Geometry: final body of the model. Coordinates: model frame, mm. A direction names the side the tool comes from. Round coordinates to 2 decimals unless told otherwise and drop trailing zeros. Loops run counter-clockwise (first coordinate to the right, second up) from the corner with the lowest first, then second, coordinate; pieces in that order, holes last. Notation, with made-up numbers: (65, 9.5) -> (114, 9.5) arc R13 cw to (114, 25.5) -> close; hole circle Ø5 at (17.25, 11). An arc over 180 degrees is marked (long way). Answer in a Markdown table with one row per item.
Autodesk Inventor part; units mm, degrees
ref_plane "YZ Plane" through (0, 0, 0) normal (1, 0, 0) x (0, 1, 0)
ref_plane "XZ Plane" through (0, 0, 0) normal (0, 1, 0) x (-1, 0, 0)
ref_plane "XY Plane" through (0, 0, 0) normal (0, 0, 1) x (1, 0, 0)
sketch "Sketch1" plane through (0, 0, 0) normal (0, 1, 0) x (-1, 0, 0)
  line L0 (-42.5, 49) -> (42.5, 49)
  line L1 (42.5, 49) -> (42.5, -49)
  line L2 (42.5, -49) -> (-42.5, -49)
  line L3 (-42.5, -49) -> (-42.5, 49)
  line L4 (-42.5, 49) -> (42.5, -49) construction
  line L5 (42.5, 49) -> (-42.5, -49) construction
  line L6 (-39, 44) -> (39, 44) construction
  line L7 (39, 44) -> (39, -44) construction
  line L8 (39, -44) -> (-39, -44) construction
  line L9 (-39, -44) -> (-39, 44) construction
  line L10 (-39, 44) -> (39, -44) construction
  line L11 (39, 44) -> (-39, -44) construction
  point P0 (0, 0)
  dimension "d0" = 85
  dimension "d1" = 98
  dimension "d2" = 78
  dimension "d3" = 88
extrude "Extrusion1" add sketch "Sketch1" along normal blind 2
hole "Hole1" at (39, 0, 44) at (39, 0, -44) at (-39, 0, -44) at (-39, 0, 44) direction (0, 1, 0) diameter 3.6 end through all
sketch "Sketch2" plane through (0, 2, 0) normal (0, 1, 0) x (1, 0, 0)
  line L0 (40, -40) -> (-40, -40)
  line L1 (-40, -40) -> (-40, 40)
  line L2 (-40, 40) -> (40, 40)
  line L3 (40, 40) -> (40, -40)
  line L4 (40, -40) -> (-40, 40) construction
  line L5 (-40, -40) -> (40, 40) construction
  point P0 (0, 0)
  dimension "d13" = 80
  dimension "d14" = 80
extrude "Extrusion2" add sketch "Sketch2" along normal blind 10
properties part number "mainboard"
Item 1: Section query D-D, the plane z = 21. Output: boundary loops of the cut face in (x, y).
Ans:
| item | result |
|---|---|
| outline | (-42.5, 0) -> (42.5, 0) -> (42.5, 2) -> (40, 2) -> (40, 12) -> (-40, 12) -> (-40, 2) -> (-42.5, 2) -> close |
Item 2: Set-up query: faces 1 (the flat face through (-1, 7, -40)), 2 (the flat face through (40, 7, -1)), 3 (the flat face through (-40, 7, 1)), 4 (the flat face through (1, 7, 40)). Return all of +Z, -Z, +X, -X, +Y, -Y with unobstructed straight access to the full face (end or side cutting, diameter ignored); none if empty.
Ans:
| item | result |
|---|---|
| face 1 | -Z, +X, -X, +Y |
| face 2 | +Z, -Z, +X, +Y |
| face 3 | +Z, -Z, -X, +Y |
| face 4 | +Z, +X, -X, +Y |
Item 3: Section query A-A, the plane z = 44. Output: boundary loops of the cut face in (x, y).
Ans:
| item | result |
|---|---|
| outline | (-42.5, 0) -> (-40.8, 0) -> (-40.8, 2) -> (-42.5, 2) -> close; (-37.2, 0) -> (37.2, 0) -> (37.2, 2) -> (-37.2, 2) -> close; (40.8, 0) -> (42.5, 0) -> (42.5, 2) -> (40.8, 2) -> close |
Item 4: Section query C-C, the plane y = 5.5. Output: boundary loops of the cut face in (x, z).
Ans:
| item | result |
|---|---|
| outline | (-40, -40) -> (40, -40) -> (40, 40) -> (-40, 40) -> close |
Item 5: First-contact query: P1, Ø4, axis at x = 4.5, y = 5, coming from the -Z side; P2, Ø2, axis at x = 26.5, z = 32.5, coming from the -Y side; P3, Ø5, axis at x = 15, y = 5, coming from the +Z side; P4, Ø5, axis at y = 6, z = 2.5, coming from the +X side. Flat tips, straight axial feed; report the tip coordinate or a pass-through.
Ans:
| item | result |
|---|---|
| P1 | z = -40 |
| P2 | y = 0 |
| P3 | z = 40 |
| P4 | x = 40 |
Item 6: Mould query, pull axis X, two halves, no side actions, for faces 5 (the cylindrical face through (-40.785, 1.014, 44.234)), 6 (the flat face through (0.2, 2, 40.2)), 7 (the flat face through (42.5, 1, -1)). Classes: released by +X, released by -X, zero draft, split by the parting line, or undercut.
Ans:
| item | result |
|---|---|
| face 5 | undercut |
| face 6 | zero draft |
| face 7 | released by +X |
Item 7: Ray query, L1, parallel to Z at x = 39, y = 1.4; L2, parallel to X at y = 0.95, z = 44; L3, parallel to Z at x = -8, y = 11.25. Return the intervals inside material, ascending.
Ans:
| item | result |
|---|---|
| L1 | -49 to -45.8, -42.2 to 42.2, 45.8 to 49 |
| L2 | -42.5 to -40.8, -37.2 to 37.2, 40.8 to 42.5 |
| L3 | -40 to 40 |
Item 8: Section query B-B, the plane x = 4. Output: boundary loops of the cut face in (y, z).
Ans:
| item | result |
|---|---|
| outline | (0, -49) -> (2, -49) -> (2, -40) -> (12, -40) -> (12, 40) -> (2, 40) -> (2, 49) -> (0, 49) -> close |
